from build123d import *

# Parameters (mm, degrees)
SKETCH_5_W          = 58
SKETCH_5_H          = 40
EXTRUDE_3_DEPTH     = 6
SKETCH_6_W          = 8
SKETCH_6_H          = 9.5
EXTRUDE_4_DEPTH     = 6
CUT_EXTRUDE_2_REACH = 137.835
SKETCH_7_R          = 0.5
FILLET_4_R          = 4
FILLET_5_R          = 4


with BuildPart() as part:
    # Эскиз5 → Бобышка-Вытянуть3 (new body)
    with BuildSketch(Plane(origin=(0, 0, 0), x_dir=(1, 0, 0), z_dir=(0, 1, 0))):
        with Locations((-100.673147531, 130.465154765)):
            Rectangle(SKETCH_5_W, SKETCH_5_H)
    extrude(amount=EXTRUDE_3_DEPTH)

    # Эскиз6 → Бобышка-Вытянуть4 (add)
    with BuildSketch(Plane.XZ):
        with Locations((-75.673147531, -115.215154765)):
            Rectangle(SKETCH_6_W, SKETCH_6_H)
        with Locations((-75.673147531, -145.715154765)):
            Rectangle(SKETCH_6_W, SKETCH_6_H)
    extrude(amount=EXTRUDE_4_DEPTH)

    # Вырез-Вытянуть2: up to this face of the body (flat: up to its plane)
    cut_extrude_2_end = Plane(part.part.faces().sort_by_distance((-97.642844501, 2.272727273, -150.465154765))[0])
    # Эскиз7 → Вырез-Вытянуть2 (cut, up to the picked face)
    with BuildSketch(Plane.XY.offset(-110.465154765), mode=Mode.PRIVATE) as cut_extrude_2_sk1:
        with Locations((-75.673147531, -3)):
            Circle(SKETCH_7_R)
    cut_extrude_2_tool1 = split(extrude(cut_extrude_2_sk1.sketch, amount=-CUT_EXTRUDE_2_REACH, mode=Mode.PRIVATE), bisect_by=cut_extrude_2_end, keep=Keep.BOTH, mode=Mode.PRIVATE)
    add(cut_extrude_2_tool1.solids().sort_by(Axis((-75.673148, -3, -110.465155), (0, 0, -1)))[0], mode=Mode.SUBTRACT)

    # Скругление4
    fillet_4_edges = [part.edges().sort_by_distance(p)[0] for p in [
        (-71.673147531, 6, -130.465154765),
        (-71.673147531, -6, -145.715154765),
        (-79.673147531, -6, -145.715154765),
        (-71.673147531, -6, -115.215154765),
        (-79.673147531, -6, -115.215154765),
    ]]
    fillet(fillet_4_edges, radius=FILLET_4_R - 0.0001)  # a hair under: the kernel refuses the full size

    # Скругление5
    fillet_5_edges = [part.edges().sort_by_distance(p)[0] for p in [
        (-129.673147531, 6, -130.465154765),
        (-129.673147531, 3, -110.465154765),
        (-129.673147531, 3, -150.465154765),
    ]]
    fillet(fillet_5_edges, radius=FILLET_5_R)


solid = part.part
Check sheet for the modelled part. Datum: model origin and axes. Units: mm. A direction names the side the tool comes from. Round coordinates to 2 decimals unless told otherwise and drop trailing zeros. Order: outer loops, then holes, each group sorted by start corner. A loop starts at its lowest first (then second) coordinate and runs counter-clockwise, first axis right, second up.
(1) Access from +Z, -Z, +X, -X, +Y, -Y to the whole of each face (thin tool, end or side, straight path). Record for faces 1 (the flat face through (-79.673, -1, -115)), 2 (the cylindrical face through (-128.53, 4.8, -130.75)), 3 (the flat face through (-76, -2, -140.965)).
(2) Scan lines: probe 1 along Z at (x, y) = (-77, -4.25); probe 2 along Y at (x, z) = (-104.5, -132.5); probe 3 along X at (y, z) = (-5.5, -147.5). Record each from-to range of solid material in increasing order.
(3) Cross-section at A-A, the plane z = -132.5. Enter the section's corners in (x, y), and give its area (3 significant figures).
(4) Go/stop test with flat-tipped pins: P1, Ø2, axis at x = -99.5, z = -144.5, coming from the -Y side; P2, Ø1, axis at y = -1.5, z = -146, coming from the -X side. Record where each tip stops, or that it passes through.
(5) Draft check along Z on faces 4 (the flat face through (-99, 3, -110.465)), 5 (the flat face through (-76, -2, -119.965)), 6 (the flat face through (-99, 3, -150.465)), 7 (the cylindrical face through (-78.53, -4.8, -145.65)). Enter one of: pulls with the +Z half, pulls with the -Z half, needs draft (parallel to the pull), parting line crosses it, or undercut.
(6) Cross-section at C-C, the plane y = 5. Enter the section's corners in (x, z).
(7) Cross-section at B-B, the plane x = -116.5. Enter the section's corners in (y, z).
Check sheet entries:
1. face 1: +Z, -Z, -X, -Y
1. face 2: +Z, -Z, -X, +Y
1. face 3: +X, -X, -Y
2. probe 1: z = -150.47 to -140.97, -119.97 to -110.47
2. probe 2: y = 0 to 6
2. probe 3: x = -77.61 to -73.74
3. outline: (-129.67, 0) - (-71.67, 0) - (-71.67, 2) arc R4 ccw to (-75.67, 6) - (-125.67, 6) arc R4 ccw to (-129.67, 2) - close
3. area: 341 mm2
4. P1: stops at y = 0
4. P2: stops at x = -79.67
5. face 4: pulls with the +Z half
5. face 5: undercut
5. face 6: pulls with the -Z half
5. face 7: needs draft
6. outline: (-128.32, -149.47) arc R4 ccw to (-125.67, -150.47) - (-73.03, -150.47) - (-73.03, -110.47) - (-125.67, -110.47) arc R4 ccw to (-128.32, -111.47) - close
7. outline: (0, -150.47) - (6, -150.47) - (6, -110.47) - (0, -110.47) - close
